Geometry check sheet. Reference: the model listing, model coordinates, mm. A direction names the side the tool comes from. Give positions to 0.01 mm unless a question says otherwise; leave off trailing zeros. Write each loop counter-clockwise with the first axis right and the second up, starting at its lowest first coordinate (ties: lowest second). Pieces come first, ordered by that corner, then holes.
(1) Cross-section at B-B (z = 25). Record the boundary of the cut face in (x, y).
(2) Mould release check, pull along Z, two halves, no side actions. Record for faces 4 (the cylindrical face through (-26, -10.8, -43.57)), 5 (the flat face through (0, 0, 1)), 6 (the flat face through (27.5, -11, -1)): +Z half, -Z half, draft (parallel to the pull), parting line (faces both ways), or undercut.
(3) Cross-section at C-C (z = -33). Record the boundary of the cut face in (x, y), and give its area (3 significant figures).
(4) Depth check by flat-ended pin: P1, Ø3.5, axis at x = 23.5, y = 1, coming from the +Z side; P2, Ø15, axis at x = 8, z = -0.5, coming from the -Y side. Enter the tip coordinate at first touch or a pass-through.
(5) Tool access check on faces 1 (the flat face through (0, 3, 1)), 2 (the flat face through (-25, -12, 0)), 3 (the flat face through (20.273, 1, 0)). Record the directions out of +Z, -Z, +X, -X, +Y, -Y that give a thin tool (end or side, any length) a straight path to the whole face; none if there is none.
(6) Cross-section at A-A (y = -22.75). Record the boundary of the cut face in (x, z).
(7) Cross-section at D-D (x = 3). Record the boundary of the cut face in (y, z), and give its area (3 significant figures).
(8) Thickness scan on line 1 along Z through (x, y) = (-1.5, -23.5); line 2 along X through (y, z) = (-7.25, 9); line 3 along Y through (x, z) = (11.5, 38.5). Record the ranges inside material, lowest first.
Autodesk Inventor part; units mm, degrees
ref_plane "YZ Plane" through (0, 0, 0) normal (1, 0, 0) x (0, 1, 0)
ref_plane "XZ Plane" through (0, 0, 0) normal (0, 1, 0) x (-1, 0, 0)
ref_plane "XY Plane" through (0, 0, 0) normal (0, 0, 1) x (1, 0, 0)
sketch "Sketch1" plane through (0, 0, 0) normal (0, 1, 0) x (-1, 0, 0)
  line L0 (22.5, 45) -> (-22.5, 45)
  line L1 (-27.5, 40) -> (-27.5, -40)
  line L2 (-22.5, -45) -> (22.5, -45)
  line L3 (27.5, -40) -> (27.5, 40)
  line L4 (27.5, 45) -> (-27.5, -45) construction
  line L5 (-27.5, 45) -> (27.5, -45) construction
  line L6 (0, 0) -> (17.6777, 17.6777) construction
  line L7 (0, 0) -> (25, 0) construction
  circle A0 centre (17.6777, 17.6777) radius 1
  line L8 (17.6777, 17.6777) -> (21.2132, 14.1421) construction
  arc A1 (21.2132, 14.1421) -> (14.1421, 21.2132) centre (17.6777, 17.6777) ccw construction
  circle A2 centre (0, 0) radius 20 construction
  line L9 (14.1421, 21.2132) -> (10.1575, 17.2286) construction
  arc A3 (-6.25, 18.9984) -> (6.25, 18.9984) centre (0, 0) ccw construction
  line L10 (21.2132, 14.1421) -> (17.2286, 10.1575) construction
  line L11 (-14.1421, 21.2132) -> (-10.1575, 17.2286) construction
  arc A4 (-14.1421, 21.2132) -> (-21.2132, 14.1421) centre (-17.6777, 17.6777) ccw construction
  line L12 (-21.2132, 14.1421) -> (-17.2286, 10.1575) construction
  circle A5 centre (-17.6777, 17.6777) radius 1
  line L13 (-21.2132, -14.1421) -> (-17.2286, -10.1575) construction
  arc A6 (-21.2132, -14.1421) -> (-14.1421, -21.2132) centre (-17.6777, -17.6777) ccw construction
  line L14 (-14.1421, -21.2132) -> (-10.1575, -17.2286) construction
  circle A7 centre (-17.6777, -17.6777) radius 1
  line L15 (14.1421, -21.2132) -> (10.1575, -17.2286) construction
  arc A8 (14.1421, -21.2132) -> (21.2132, -14.1421) centre (17.6777, -17.6777) ccw construction
  line L16 (21.2132, -14.1421) -> (17.2286, -10.1575) construction
  circle A9 centre (17.6777, -17.6777) radius 1
  line L17 (-20.273, 10) -> (-25.273, 10)
  line L18 (-25.273, 10) -> (-25.273, -10)
  line L19 (-25.273, -10) -> (-20.273, -10)
  line L20 (-20.273, -10) -> (-20.273, 10)
  line L21 (-20.273, 10) -> (-25.273, -10) construction
  line L22 (-25.273, 10) -> (-20.273, -10) construction
  line L23 (39.9497, 0) -> (-39.9497, 0)
  arc A10 (22.5, -45) -> (27.5, -40) centre (22.5, -40) ccw
  arc A11 (27.5, 40) -> (22.5, 45) centre (22.5, 40) ccw
  arc A12 (-22.5, 45) -> (-27.5, 40) centre (-22.5, 40) ccw
  arc A13 (-27.5, -40) -> (-22.5, -45) centre (-22.5, -40) ccw
  point P0 (-22.773, 0)
  point P1 (-22.773, 0)
  dimension "d0" = 55
  dimension "d1" = 90
  dimension "d4" = 25
  dimension "d5" = 45
  dimension "d6" = 2
  dimension "d7" = 5
  dimension "d8" = 360
  dimension "d9" = 5
  dimension "d10" = 20
  dimension "d18" = 5
extrude "Extrusion1" add sketch "Sketch1" along normal blind 3 contours A11 L3 L23 L20 L17 L18 L1 A12 L0 | L3 A10 L2 A13 L1 L23 L18 L19 L20
sketch "Sketch2" plane through (0, 0, 0) normal (0, -1, 0) x (1, 0, 0)
  line L0 (22.5, 45) -> (-22.5, 45)
  line L1 (-27.5, 40) -> (-27.5, -40)
  line L2 (-22.5, -45) -> (22.5, -45)
  line L3 (27.5, -40) -> (27.5, 40)
  line L4 (27.5, 45) -> (-27.5, -45) construction
  line L5 (-27.5, 45) -> (27.5, -45) construction
  line L6 (17, 42.5) -> (-17, 42.5)
  line L7 (-25, 34.5) -> (-25, -34.5)
  line L8 (-17, -42.5) -> (17, -42.5)
  line L9 (25, -34.5) -> (25, 34.5)
  line L10 (25, 42.5) -> (-25, -42.5) construction
  line L11 (-25, 42.5) -> (25, -42.5) construction
  arc A0 (25, 34.5) -> (17, 42.5) centre (17, 34.5) ccw
  arc A1 (17, -42.5) -> (25, -34.5) centre (17, -34.5) ccw
  arc A2 (-25, -34.5) -> (-17, -42.5) centre (-17, -34.5) ccw
  arc A3 (-17, 42.5) -> (-25, 34.5) centre (-17, 34.5) ccw
  arc A4 (27.5, 40) -> (22.5, 45) centre (22.5, 40) ccw
  arc A5 (-22.5, 45) -> (-27.5, 40) centre (-22.5, 40) ccw
  arc A6 (-27.5, -40) -> (-22.5, -45) centre (-22.5, -40) ccw
  arc A7 (22.5, -45) -> (27.5, -40) centre (22.5, -40) ccw
  point P0 (0, 0)
  dimension "d13" = 55
  dimension "d14" = 90
  dimension "d15" = 50
  dimension "d16" = 85
  dimension "d17" = 8
  dimension "d21" = 5
extrude "Extrusion2" add sketch "Sketch2" along normal blind 25
sketch "Sketch3" plane through (27.5, 3, 40) normal (1, 0, 0) x (0, 0, -1)
  circle A0 centre (10.9293, -14.3731) radius 5
  point P0 (40, -3)
  dimension "d22" = 10
extrude "Extrusion3" cut sketch "Sketch3" against normal up to surface (2.5 mm away)
properties part number "mount1"
Reply:
1. outline: (-27.5, -25) - (-25, -25) - (-25, 0) - (25, 0) - (25, -8.47) - (27.5, -8.47) - (27.5, 3) - (-27.5, 3) - close; (25, -25) - (27.5, -25) - (27.5, -14.28) - (25, -14.28) - close
2. face 4: -Z half
2. face 5: undercut
2. face 6: draft
3. outline: (-27.5, -25) - (-25, -25) - (-25, 0) - (25, 0) - (25, -25) - (27.5, -25) - (27.5, 3) - (-27.5, 3) - close
3. area: 290 mm2
4. P1: stops at z = 45
4. P2: stops at y = 0
5. face 1: +Z, -Z, +X, -X, +Y
5. face 2: -Y
5. face 3: +Y, -Y
6. outline: (-27.5, -40) arc R5 ccw to (-22.5, -45) - (22.5, -45) arc R5 ccw to (27.5, -40) - (27.5, 40) arc R5 ccw to (22.5, 45) - (-22.5, 45) arc R5 ccw to (-27.5, 40) - close; hole (-25, -34.5) arc R8 ccw to (-17, -42.5) - (17, -42.5) arc R8 ccw to (25, -34.5) - (25, 34.5) arc R8 ccw to (17, 42.5) - (-17, 42.5) arc R8 ccw to (-25, 34.5) - close
7. outline: (-25, -45) - (3, -45) - (3, 45) - (-25, 45) - (-25, 42.5) - (0, 42.5) - (0, -42.5) - (-25, -42.5) - close
7. area: 395 mm2
8. line 1: z = -45 to -42.5, 42.5 to 45
8. line 2: x = -27.5 to -25, 25 to 27.5
8. line 3: y = 0 to 3
